Source: CAD feature listing. Evaluate the final solid. Frame: model axes, mm. A direction names the side the tool comes from. Round coordinates to 2 decimals unless told otherwise and drop trailing zeros. Loops run counter-clockwise (first coordinate to the right, second up) from the corner with the lowest first, then second, coordinate; pieces in that order, holes last.
Item 1: Section query A-A on z = 6.25. Return loops of the section in (x, y).
Item 2: Ray query, L1, parallel to Y at x = -7.5, z = 7.75; L2, parallel to Z at x = 18.5, y = 15. Return the intervals inside material, ascending.
Item 3: Pull-direction query (X, two-part tool) for faces 5 (the flat face through (4, -8, 6)), 6 (the flat face through (-7, 7, 8)), 7 (the flat face through (5, 6.5, 6)), 8 (the flat face through (18.99, -19.05, 1.97)); classes: released by +X, released by -X, zero draft, split by the parting line, or undercut.
Item 4: First-contact query: P1, Ø0.8, axis at x = -8, z = 5, coming from the +Y side; P2, Ø1.1, axis at x = -22.5, z = 2, coming from the -Y side; P3, Ø1.8, axis at x = 23.5, z = 2, coming from the +Y side. Flat tips, straight axial feed; report the tip coordinate or a pass-through.
Item 5: Access query for faces 1 (the flat face through (-6, 9, 6)), 2 (the flat face through (9, 7, 6)), 3 (the flat face through (-6.5, -5, 6)), 4 (the flat face through (23, 16.8, 2)). Directions: +Z, -Z, +X, -X, +Y, -Y. A direction counts if a zero-diameter tool reaches every point of the face in a straight line with its end or side. Return the directions, or none.
Item 6: Section query C-C on z = 1.75. Return loops of the section in (x, y).
Item 7: Section query D-D on y = 10.5. Return loops of the section in (x, z), then the cut area to 3 significant figures.
Item 8: Section query B-B on x = 8. Return loops of the section in (y, z), then the cut area to 3 significant figures.
Autodesk Inventor part; units mm, degrees
ref_plane "YZ Plane" through (0, 0, 0) normal (1, 0, 0) x (0, 1, 0)
ref_plane "XZ Plane" through (0, 0, 0) normal (0, 1, 0) x (-1, 0, 0)
ref_plane "XY Plane" through (0, 0, 0) normal (0, 0, 1) x (1, 0, 0)
sketch "草图1" plane through (0, 0, 0) normal (0, 0, 1) x (1, 0, 0)
  line L0 (24.9, 0) -> (24.9, 16.8)
  line L1 (24.9, 16.8) -> (21.24, 16.8)
  line L2 (21.24, 16.8) -> (16.7994, 21.2406)
  line L3 (16.7994, 21.2406) -> (16.7994, 24.9006)
  line L4 (16.7994, 24.9006) -> (-0.0006, 24.9006)
  line L5 (-0.0006, 24.9006) -> (-16.8006, 24.9006)
  line L6 (-16.8006, 24.9006) -> (-16.8006, 21.2406)
  line L7 (-16.8006, 21.2406) -> (-21.2413, 16.8)
  line L8 (-21.2413, 16.8) -> (-24.9013, 16.8)
  line L9 (-24.9013, 16.8) -> (-24.9013, 0)
  line L10 (-24.9013, 0) -> (-24.9013, -16.8)
  line L11 (-24.9013, -16.8) -> (-21.2413, -16.8)
  line L12 (-21.2413, -16.8) -> (-16.8006, -21.2406)
  line L13 (-16.8006, -21.2406) -> (-16.8006, -24.9006)
  line L14 (-16.8006, -24.9006) -> (-0.0006, -24.9006)
  line L15 (-0.0006, -24.9006) -> (16.7994, -24.9006)
  line L16 (16.7994, -24.9006) -> (16.7994, -21.2406)
  line L17 (16.7994, -21.2406) -> (21.24, -16.8)
  line L18 (21.24, -16.8) -> (24.9, -16.8)
  line L19 (24.9, -16.8) -> (24.9, 0)
  point P0 (0, 0)
extrude "拉伸1" add sketch "草图1" along normal blind 4
sketch "草图2" plane through (0, 0, 4) normal (0, 0, 1) x (1, 0, 0)
  line L0 (-6.5, -6.5) -> (6.5, -6.5)
  line L1 (6.5, -6.5) -> (6.5, 6.5)
  line L2 (6.5, 6.5) -> (-6.5, 6.5)
  line L3 (-6.5, 6.5) -> (-6.5, -6.5)
  line L4 (-6.5, -6.5) -> (6.5, 6.5) construction
  line L5 (6.5, -6.5) -> (-6.5, 6.5) construction
  line L6 (-6.5, -6.5) -> (6.5, -6.5) construction
  line L7 (-6.5, 6.5) -> (-4.5, 6.5)
  line L8 (-9, 4) -> (-4, 4)
  line L9 (-4, 4) -> (-4, 9)
  line L10 (-4, 9) -> (-9, 9)
  line L11 (-9, 9) -> (-9, 4)
  line L12 (-9, 4) -> (-4, 9) construction
  line L13 (-4, 4) -> (-9, 9) construction
  line L14 (9, 4) -> (4, 4)
  line L15 (4, 4) -> (4, 9)
  line L16 (4, 9) -> (9, 9)
  line L17 (9, 9) -> (9, 4)
  line L18 (9, 4) -> (4, 9) construction
  line L19 (4, 4) -> (9, 9) construction
  line L20 (-9, -9) -> (-4, -9)
  line L21 (-4, -9) -> (-4, -4)
  line L22 (-4, -4) -> (-9, -4)
  line L23 (-9, -4) -> (-9, -9)
  line L24 (-9, -9) -> (-4, -4) construction
  line L25 (-4, -9) -> (-9, -4) construction
  line L26 (4, -4) -> (9, -4)
  line L27 (9, -4) -> (9, -9)
  line L28 (9, -9) -> (4, -9)
  line L29 (4, -9) -> (4, -4)
  line L30 (4, -4) -> (9, -9) construction
  line L31 (9, -4) -> (4, -9) construction
  point P0 (0, 0)
  point P1 (-4, -6.5)
  point P2 (-6.5, -4)
  point P3 (6.5, -4)
  point P4 (4, -6.5)
  point P5 (4, 6.5)
  point P6 (6.5, 4)
  point P7 (-6.5, 4)
  point P8 (-4, 6.5)
extrude "拉伸2" add sketch "草图2" along normal blind 4 contours L0 L21 L20 L23 L22 L3 | L0 L1 L26 L27 L28 L29 | L8 L11 L10 L9 L2 L3 | L1 L2 L15 L16 L17 L14
equation "\"BendRadius\" = Thickness"
equation "\"BendReliefWidth\" = Thickness"
equation "\"BendReliefDepth\" = 0.5 * Thickness"
equation "\"CornerReliefSize\" = 4 * Thickness"
equation "\"MinimumRemnant\" = 2 * Thickness"
equation "\"TransitionRadius\" = BendRadius"
equation "\"JacobiRadiusSize\" = BendRadius"
equation "\"GapSize\" = Thickness"
properties part number "样品池"
Data:
1. outline: (-9, -9) - (-4, -9) - (-4, -6.5) - (-6.5, -6.5) - (-6.5, -4) - (-9, -4) - close; (-9, 4) - (-6.5, 4) - (-6.5, 6.5) - (-4, 6.5) - (-4, 9) - (-9, 9) - close; (4, -9) - (9, -9) - (9, -4) - (6.5, -4) - (6.5, -6.5) - (4, -6.5) - close; (4, 6.5) - (6.5, 6.5) - (6.5, 4) - (9, 4) - (9, 9) - (4, 9) - close
2. L1: y = -9 to -4, 4 to 9
2. L2: z = 0 to 4
3. face 5: undercut
3. face 6: zero draft
3. face 7: undercut
3. face 8: released by +X
4. P1: stops at y = 9
4. P2: stops at y = -16.8
4. P3: stops at y = 16.8
5. face 1: +Z, +X, -X, +Y
5. face 2: +Z, +X, +Y, -Y
5. face 3: +Z
5. face 4: +Z, -Z, +X, +Y
6. outline: (-24.9, -16.8) - (-21.24, -16.8) - (-16.8, -21.24) - (-16.8, -24.9) - (16.8, -24.9) - (16.8, -21.24) - (21.24, -16.8) - (24.9, -16.8) - (24.9, 16.8) - (21.24, 16.8) - (16.8, 21.24) - (16.8, 24.9) - (-16.8, 24.9) - (-16.8, 21.24) - (-21.24, 16.8) - (-24.9, 16.8) - close
7. outline: (-24.9, 0) - (24.9, 0) - (24.9, 4) - (-24.9, 4) - close
7. area: 199 mm2
8. outline: (-24.9, 0) - (24.9, 0) - (24.9, 4) - (9, 4) - (9, 8) - (4, 8) - (4, 4) - (-4, 4) - (-4, 8) - (-9, 8) - (-9, 4) - (-24.9, 4) - close
8. area: 239 mm2
